from build123d import *

# Parameters (mm, degrees)
SKETCH_1_R      = 15
SKETCH_1_R_2    = 10
EXTRUDE_1_DEPTH = 30
SKETCH_2_R      = 20
SKETCH_2_R_2    = 15
SKETCH_2_R_3    = 10
EXTRUDE_2_DEPTH = 5
F_3_0MM_1_D     = 3
F_3_0MM_1_DEPTH = 7.5
F_3_0MM_1_TIP   = 0.901290929


with BuildPart() as part:
    # 草图1 → 凸台-拉伸1 (new body)
    with BuildSketch(Plane(origin=(0, 0, 0), x_dir=(1, 0, 0), z_dir=(0, 1, 0))):
        with Locations(Location((0, 0, 0), (0, 0, 270))):
            Circle(SKETCH_1_R)
        with Locations(Location((0, 0, 0), (0, 0, 270))):
            Circle(SKETCH_1_R_2, mode=Mode.SUBTRACT)
    extrude(amount=EXTRUDE_1_DEPTH)

    # 草图2 → 凸台-拉伸2 (add)
    # profile 1 of 2: a face of its own
    with BuildSketch(Plane(origin=(0, 30, 0), x_dir=(1, 0, 0), z_dir=(0, 1, 0))):
        with Locations(Location((0, 0, 0), (0, 0, 270))):
            Circle(SKETCH_2_R)
        with Locations(Location((0, 0, 0), (0, 0, 270))):
            Circle(SKETCH_2_R_2, mode=Mode.SUBTRACT)
    # profile 2 of 2: a face of its own
    with BuildSketch(Plane(origin=(0, 30, 0), x_dir=(1, 0, 0), z_dir=(0, 1, 0))):
        with Locations(Location((0, 0, 0), (0, 0, 270))):
            Circle(SKETCH_2_R_2)
        with Locations(Location((0, 0, 0), (0, 0, 270))):
            Circle(SKETCH_2_R_3, mode=Mode.SUBTRACT)
    extrude(amount=EXTRUDE_2_DEPTH)

    # Ø3.0mm 暗销孔1
    with Locations(Plane(origin=(0, 35, 0), x_dir=(1, 0, 0), z_dir=(0, 1, 0))):
        with Locations((0, 17.5), (17.5, 0), (0, -17.5), (-17.5, 0)):
            Hole(F_3_0MM_1_D / 2, depth=F_3_0MM_1_DEPTH)
            with Locations((0, 0, -(F_3_0MM_1_DEPTH + F_3_0MM_1_TIP / 2))):  # 118° drill point
                Cone(0, F_3_0MM_1_D / 2, F_3_0MM_1_TIP, mode=Mode.SUBTRACT)


solid = part.part
Verification items for the finished model (mm, model axes). A direction names the side the tool comes from. Give positions to 0.01 mm unless a question says otherwise; leave off trailing zeros. Order: outer loops, then holes, each group sorted by start corner. A loop starts at its lowest first (then second) coordinate and runs counter-clockwise, first axis right, second up. Notation, with made-up numbers: M 62,63.5 L 73,63.5 A18 ccw 73,93.5 Z; hole C -31.5,64.5 d6. An arc over 180 degrees is marked long. Use one line per item in the form item = value. Start each with the question number.
Q1. Section check B-B (x = 0). Enter the section's corners in (y, z).
Q2. Access from +Z, -Z, +X, -X, +Y, -Y to the whole of each face (thin tool, end or side, straight path). Record for faces 4 (the flat face through (-13, 30, -8)), 5 (the cylindrical face through (-16, 32, 0)).
Q3. Go/stop test with flat-tipped pins: pin 1 Ø3.5 at (x, z) = (0, 17.5) entering from +Y; pin 2 Ø4 at (y, z) = (26.5, -7.5) entering from +X; pin 3 Ø1.5 at (x, z) = (8.5, 2) entering from -Y; pin 4 Ø3 at (x, y) = (-10, 22.5) entering from -Z. Record where each tip stops, or that it passes through.
Q4. Section check D-D (x = 17.5). Enter the section's corners in (y, z).
Q5. Section check C-C (z = -17.5). Enter the section's corners in (x, y).
Q6. Mould release check, pull along X, two halves, no side actions. Record for faces 1 (the cylindrical face through (19, 32, 0)), 2 (the flat face through (9, 35, -5)), 3 (the cylindrical face through (0.66, 14.79, -14.985)): +X half, -X half, draft (parallel to the pull), parting line (faces both ways), or undercut.
Q7. Section check A-A (z = 0). Enter the section's corners in (x, y), then the cut area to 3 significant figures.
Q8. Scan lines: line 1 along Y through (x, z) = (-6, 16); line 2 along Z through (x, y) = (9, 11); line 3 along Z through (x, y) = (17.5, 33.55). Record each from-to range of solid material in increasing order. Write a range as [from, to].
Evaluation:
q1.outline = M 0,-15 L 30,-15 L 30,-16 L 35,-16 L 35,-10 L 0,-10 Z; M 0,10 L 35,10 L 35,16 L 30,16 L 30,15 L 0,15 Z; M 30,-20 L 35,-20 L 35,-19 L 30,-19 Z; M 30,19 L 35,19 L 35,20 L 30,20 Z
q2.face_4 = -Y
q2.face_5 = +Y, -Y
q3.pin_1 = 35
q3.pin_2 = 13.96
q3.pin_3 = through
q3.pin_4 = -12.36
q4.outline = M 30,-9.68 L 35,-9.68 L 35,-1.5 L 30,-1.5 Z; M 30,1.5 L 35,1.5 L 35,9.68 L 30,9.68 Z
q5.outline = M -9.68,30 L -1.5,30 L -1.5,35 L -9.68,35 Z; M 1.5,30 L 9.68,30 L 9.68,35 L 1.5,35 Z
q6.face_1 = undercut
q6.face_2 = draft
q6.face_3 = parting line
q7.outline = M -20,30 L -19,30 L -19,35 L -20,35 Z; M -16,30 L -15,30 L -15,0 L -10,0 L -10,35 L -16,35 Z; M 10,0 L 15,0 L 15,30 L 16,30 L 16,35 L 10,35 Z; M 19,30 L 20,30 L 20,35 L 19,35 Z
q7.area = 370 mm2
q8.line_1 = [30, 35]
q8.line_2 = [-12, -4.36], [4.36, 12]
q8.line_3 = [-9.68, -1.5], [1.5, 9.68]
